Source: CAD feature listing. Evaluate the final solid. Frame: model axes, mm. Face numbers are marked on the shaded views. A direction names the side the tool comes from. Coordinates: 2 decimals unless noted, no trailing zeros. Order: outer loops, then holes, each group sorted by start corner. A loop starts at its lowest first (then second) coordinate and runs counter-clockwise, first axis right, second up. Notation, with made-up numbers: (-29, 19.5) - (2, 19.5) arc R20 ccw to (2, 24.5) - close; hole circle Ø10 at (-26.75, 85). An arc over 180 degrees is marked (long way). One line per question, with ' | ' between items.
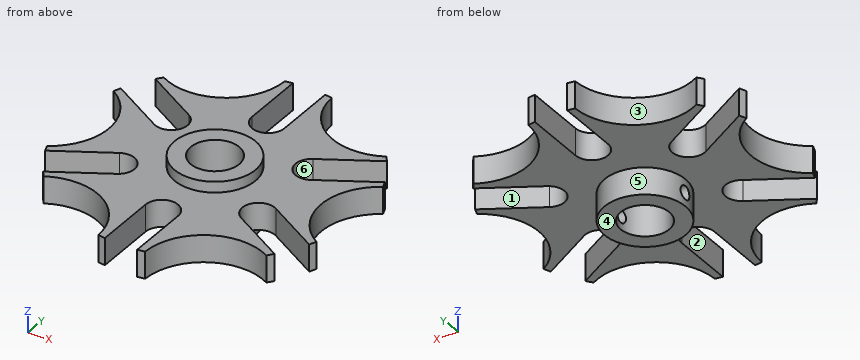
from build123d import *

# Parameters (mm, degrees)
FORO_7_5_7_5_1_D         = 7.5
SCHIZZO9_OUTSIDE_W       = 207.824
SCHIZZO9_OUTSIDE_H       = 207.824
TAGLIO_ESTRUSIONE1_DEPTH = 116.069544208


with BuildPart() as part:
    # Schizzo6 → Rivoluzione1 (revolve)
    with BuildSketch(Plane(origin=(0, 0, 0), x_dir=(1, 0, 0), z_dir=(0, 1, 0)), mode=Mode.PRIVATE) as rivoluzione1_sk:
        Polygon((13.5, 0), (13.5, 36), (22.5, 36), (22.5, 21), (80, 21), (80, 6), (22.5, 6), (22.5, 0), align=None)
    revolve(rivoluzione1_sk.sketch.rotate(Axis((0, 0, -47.894415312), (0, 0, 1)), 180), axis=Axis((0, 0, -47.894415312), (0, 0, 1)))

    # Foro Ø7.5 (7.5)-1 (through all)
    with Locations(Plane(origin=(22.5, 0, 0), x_dir=(0, 0, -1), z_dir=(1, 0, 0))):
        with Locations((28.5, 0)):
            Hole(FORO_7_5_7_5_1_D / 2)

    # Schizzo9 outside → Taglio-Estrusione1 (cut, through all)
    with BuildSketch(Plane(origin=(0, 0, -21), x_dir=(-1, 0, 0), z_dir=(0, 0, -1))):
        Rectangle(SCHIZZO9_OUTSIDE_W, SCHIZZO9_OUTSIDE_H)
        with BuildLine():
            Line((9, 79.492137976), (9, 45))
            ThreePointArc((9, 45), (0, 36), (-9, 45))
            Line((-9, 45), (-9, 79.492137976))
            Line((-9, 79.492137976), (-13.008275981, 78.935320079))
            ThreePointArc((-13.008275981, 78.935320079), (-29.5, 51.095498823), (-61.855854454, 50.733157498))
            Line((-61.855854454, 50.733157498), (-64.342210888, 47.540297622))
            Line((-64.342210888, 47.540297622), (-34.47114317, 30.294228634))
            ThreePointArc((-34.47114317, 30.294228634), (-31.176914536, 18), (-43.47114317, 14.705771366))
            Line((-43.47114317, 14.705771366), (-73.342210888, 31.951840354))
            Line((-73.342210888, 31.951840354), (-74.864130435, 28.202162581))
            ThreePointArc((-74.864130435, 28.202162581), (-59, 0), (-74.864130435, -28.202162581))
            Line((-74.864130435, -28.202162581), (-73.342210888, -31.951840354))
            Line((-73.342210888, -31.951840354), (-43.47114317, -14.705771366))
            ThreePointArc((-43.47114317, -14.705771366), (-31.176914536, -18), (-34.47114317, -30.294228634))
            Line((-34.47114317, -30.294228634), (-64.342210888, -47.540297622))
            Line((-64.342210888, -47.540297622), (-61.855854454, -50.733157498))
            ThreePointArc((-61.855854454, -50.733157498), (-29.5, -51.095498823), (-13.008275981, -78.935320079))
            Line((-13.008275981, -78.935320079), (-9, -79.492137976))
            Line((-9, -79.492137976), (-9, -45))
            ThreePointArc((-9, -45), (0, -36), (9, -45))
            Line((9, -45), (9, -79.492137976))
            Line((9, -79.492137976), (13.008275981, -78.935320079))
            ThreePointArc((13.008275981, -78.935320079), (29.5, -51.095498823), (61.855854454, -50.733157498))
            Line((61.855854454, -50.733157498), (64.342210888, -47.540297622))
            Line((64.342210888, -47.540297622), (34.47114317, -30.294228634))
            ThreePointArc((34.47114317, -30.294228634), (31.176914536, -18), (43.47114317, -14.705771366))
            Line((43.47114317, -14.705771366), (73.342210888, -31.951840354))
            Line((73.342210888, -31.951840354), (74.864130435, -28.202162581))
            ThreePointArc((74.864130435, -28.202162581), (59, 0), (74.864130435, 28.202162581))
            Line((74.864130435, 28.202162581), (73.342210888, 31.951840354))
            Line((73.342210888, 31.951840354), (43.47114317, 14.705771366))
            ThreePointArc((43.47114317, 14.705771366), (31.176914536, 18), (34.47114317, 30.294228634))
            Line((34.47114317, 30.294228634), (64.342210888, 47.540297622))
            Line((64.342210888, 47.540297622), (61.855854454, 50.733157498))
            ThreePointArc((61.855854454, 50.733157498), (29.5, 51.095498823), (13.008275981, 78.935320079))
            Line((13.008275981, 78.935320079), (9, 79.492137976))
        make_face(mode=Mode.SUBTRACT)
    extrude(amount=-TAGLIO_ESTRUSIONE1_DEPTH, mode=Mode.SUBTRACT)


solid = part.part
(1) Cut plane A-A (y = 0). Return the cut outline in (x, z).
Taken from the geometry:
outline: (-59, -21) - (-22.5, -21) - (-22.5, -24.75) - (-13.5, -24.75) - (-13.5, 0) - (-22.5, 0) - (-22.5, -6) - (-59, -6) - close; (-22.5, -36) - (-13.5, -36) - (-13.5, -32.25) - (-22.5, -32.25) - close; (13.5, -36) - (22.5, -36) - (22.5, -32.25) - (13.5, -32.25) - close; (13.5, -24.75) - (22.5, -24.75) - (22.5, -21) - (59, -21) - (59, -6) - (22.5, -6) - (22.5, 0) - (13.5, 0) - close
(2) Pin query (flat end, axial travel): P1, Ø16.5, axis at y = 64, z = -12, coming from the -X side; P2, Ø7.5, axis at y = -68, z = -12.5, coming from the +X side; P3, Ø10, axis at x = -29.5, y = -12.5, coming from the +Z side. Return the tip coordinate at first contact, or that it passes through.
Taken from the geometry:
P1: stops at x = -23.27 | P2: stops at x = 16.83 | P3: stops at z = -6
(3) Cut plane B-B (x = 50). Return the cut outline in (y, z), and give its area (3 significant figures).
Taken from the geometry:
outline: (-46.92, -21) - (-39.26, -21) - (-39.26, -6) - (-46.92, -6) - close; (-18.48, -21) - (18.48, -21) - (18.48, -6) - (-18.48, -6) - close; (39.26, -21) - (46.92, -21) - (46.92, -6) - (39.26, -6) - close | area: 784 mm²
(4) Pull-direction query (X, two-part tool) for the marked faces 4, 5 and 6; classes: pulls with the +X half, pulls with the -X half, needs draft (parallel to the pull), parting line crosses it, or undercut.
Taken from the geometry:
face 4: needs draft | face 5: parting line crosses it | face 6: undercut
(5) Cut plane C-C (z = -28). Return the cut outline in (x, y).
Taken from the geometry:
outline: (-22.19, -3.72) arc R22.5 ccw to (22.19, -3.72) - (12.98, -3.72) arc R13.5 cw to (-12.98, -3.72) - close; (-22.19, 3.72) - (-12.98, 3.72) arc R13.5 cw to (12.98, 3.72) - (22.19, 3.72) arc R22.5 ccw to start
(6) Material intervals for L1, parallel to Y at x = -46, z = -6.5; L2, parallel to Y at x = 34, z = -15; L3, parallel to X at y = 50, z = -9.5, sorted ascending. Write a range as from..to.
Taken from the geometry:
L1: y = -46.67..-36.95, -16.17..16.17, 36.95..46.67 | L2: y = -48.93..-30, -15..15, 30..48.93 | L3: x = -62.43..-60.44, -31.56..-9, 9..31.56, 60.44..62.43
(7) Set-up query: the marked faces 1, 2 and 3. Return all of +Z, -Z, +X, -X, +Y, -Y with unobstructed straight access to the full face (end or side cutting, diameter ignored); none if empty.
Taken from the geometry:
face 1: +Z, -Z | face 2: +Z, -Z, -Y | face 3: +Z, -Z, +Y
(8) Cut plane D-D (x = -6.5). Return the cut outline in (y, z).
Taken from the geometry:
outline: (-38.78, -21) - (-21.54, -21) - (-21.54, -36) - (-11.83, -36) - (-11.83, 0) - (-21.54, 0) - (-21.54, -6) - (-38.78, -6) - close; (11.83, -36) - (21.54, -36) - (21.54, -21) - (38.78, -21) - (38.78, -6) - (21.54, -6) - (21.54, 0) - (11.83, 0) - close
